from build123d import *

# Parameters (mm, degrees)
BOSS_EXTRUDE2_DEPTH = 5
BOSS_EXTRUDE3_DEPTH = 0.5


with BuildPart() as part:
    # Sketch1 → Boss-Extrude2 (new body)
    with BuildSketch(Plane.XY):
        with BuildLine():
            Line((-5.525095111, -0.448623985), (-5.525095111, 0.021401397))
            ThreePointArc((-5.525095111, 0.021401397), (-5.407937823, 0.304244109), (-5.125095111, 0.421401397))
            Line((-5.125095111, 0.421401397), (1.074904889, 0.421401397))
            ThreePointArc((1.074904889, 0.421401397), (1.357747601, 0.304244109), (1.474904889, 0.021401397))
            Line((1.474904889, 0.021401397), (1.474904889, -0.448623985))
            ThreePointArc((1.474904889, -0.448623985), (1.442603337, -0.557606693), (1.356132582, -0.631386295))
            Line((1.356132582, -0.631386295), (-0.697525505, -1.544123223))
            ThreePointArc((-0.697525505, -1.544123223), (-0.776944296, -1.569884846), (-0.859980891, -1.578598603))
            Line((-0.859980891, -1.578598603), (-3.190209331, -1.578598603))
            ThreePointArc((-3.190209331, -1.578598603), (-3.273245926, -1.569884846), (-3.352664717, -1.544123223))
            Line((-3.352664717, -1.544123223), (-5.406322804, -0.631386295))
            ThreePointArc((-5.406322804, -0.631386295), (-5.492793559, -0.557606693), (-5.525095111, -0.448623985))
        make_face()
        with BuildLine():
            Line((-0.778753198, -1.361360913), (1.274904889, -0.448623985))
            Line((1.274904889, -0.448623985), (1.274904889, 0.021401397))
            ThreePointArc((1.274904889, 0.021401397), (1.216326245, 0.162822753), (1.074904889, 0.221401397))
            Line((1.074904889, 0.221401397), (-5.125095111, 0.221401397))
            ThreePointArc((-5.125095111, 0.221401397), (-5.266516467, 0.162822753), (-5.325095111, 0.021401397))
            Line((-5.325095111, 0.021401397), (-5.325095111, -0.448623985))
            Line((-5.325095111, -0.448623985), (-3.271437024, -1.361360913))
            ThreePointArc((-3.271437024, -1.361360913), (-3.231727628, -1.374241725), (-3.190209331, -1.378598603))
            Line((-3.190209331, -1.378598603), (-0.859980891, -1.378598603))
            ThreePointArc((-0.859980891, -1.378598603), (-0.818462594, -1.374241725), (-0.778753198, -1.361360913))
        make_face(mode=Mode.SUBTRACT)
    extrude(amount=BOSS_EXTRUDE2_DEPTH)

    # Sketch2 → Boss-Extrude3 (add)
    with BuildSketch(Plane.XY):
        with BuildLine():
            Line((-3.190209331, -1.378598603), (-0.859980891, -1.378598603))
            ThreePointArc((-0.859980891, -1.378598603), (-0.818462594, -1.374241725), (-0.778753198, -1.361360913))
            Line((-0.778753198, -1.361360913), (1.274904889, -0.448623985))
            Line((1.274904889, -0.448623985), (1.274904889, 0.304244109))
            Line((1.274904889, 0.304244109), (-5.407937823, 0.304244109))
            Line((-5.407937823, 0.304244109), (-5.407937823, -0.448623985))
            Line((-5.407937823, -0.448623985), (-5.325095111, -0.448623985))
            Line((-5.325095111, -0.448623985), (-3.271437024, -1.361360913))
            ThreePointArc((-3.271437024, -1.361360913), (-3.231727628, -1.374241725), (-3.190209331, -1.378598603))
        make_face()
    extrude(amount=BOSS_EXTRUDE3_DEPTH)


solid = part.part
Check sheet for the modelled part. Datum: model origin and axes. Units: mm. A direction names the side the tool comes from. Give positions to 0.01 mm unless a question says otherwise; leave off trailing zeros. Loops run counter-clockwise (first coordinate to the right, second up) from the corner with the lowest first, then second, coordinate; pieces in that order, holes last. Notation, with made-up numbers: M -34,35.5 L 1,35.5 A17 ccw 1,42.5 Z; hole C -6.75,13.5 d3. An arc over 180 degrees is marked long. Answer as a JSON object with one key per item and string values. Group by question number.
Q1. Cross-section at B-B on y = -0.3. Record the cut outline in (x, z), then the cut area to 3 significant figures.
Q2. Release check for a two-part mould opening along X. For faces 3 (the flat face through (-4.31, -0.9, 2.72)), 4 (the flat face through (0.3, -1.1, 2.5)), 5 (the flat face through (-2, -1.579, 2)) record: released by +X, released by -X, zero draft, split by the parting line, or undercut.
Q3. Cross-section at C-C on x = -3. Record the cut outline in (y, z).
Q4. Material ranges on line 1 along Y through (x, z) = (-1.5, 4.1); line 2 along X through (y, z) = (-0.3, 3.95); line 3 along Z through (x, y) = (-4.25, -0.35), recorded low to high. Write a range as [from, to].
Q5. Cross-section at A-A on z = 3.15. Record the cut outline in (x, y).
Q6. Access from +Z, -Z, +X, -X, +Y, -Y to the whole of each face (thin tool, end or side, straight path). Record for faces 1 (the flat face through (-4.37, -1.09, 2.46)), 2 (the flat face through (-2, 0, 0.5)).
Evaluation:
{
 "1": {"outline": "M -5.53,0 L 1.47,0 L 1.47,5 L 1.27,5 L 1.27,0.5 L -5.33,0.5 L -5.33,5 L -5.53,5 Z", "area": "5.30 mm2"},
 "2": {"face 3": "undercut", "face 4": "released by +X", "face 5": "zero draft"},
 "3": {"outline": "M -1.58,0 L 0.42,0 L 0.42,5 L 0.22,5 L 0.22,0.5 L -1.38,0.5 L -1.38,5 L -1.58,5 Z"},
 "4": {"line 1": "y = [-1.58, -1.38], [0.22, 0.42]", "line 2": "x = [-5.53, -5.33], [1.27, 1.47]", "line 3": "z = [0, 0.5]"},
 "5": {"outline": "M -5.53,-0.45 A0.2 ccw -5.41,-0.63 L -3.35,-1.54 A0.4 ccw -3.19,-1.58 L -0.86,-1.58 A0.4 ccw -0.7,-1.54 L 1.36,-0.63 A0.2 ccw 1.47,-0.45 L 1.47,0.02 A0.4 ccw 1.07,0.42 L -5.13,0.42 A0.4 ccw -5.53,0.02 Z; hole M -5.33,-0.45 L -3.27,-1.36 A0.2 ccw -3.19,-1.38 L -0.86,-1.38 A0.2 ccw -0.78,-1.36 L 1.27,-0.45 L 1.27,0.02 A0.2 ccw 1.07,0.22 L -5.13,0.22 A0.2 ccw -5.33,0.02 Z"},
 "6": {"face 1": "+Z, -Z, -X, -Y", "face 2": "+Z"}
}
